Job drawing, mm, ordinate dimensions from the low corner. One solid piece. A direction names the side the tool comes from. Give positions to 0.01 mm unless a question says otherwise; leave off trailing zeros. Write each loop counter-clockwise with the first axis right and the second up, starting at its lowest first coordinate (ties: lowest second). Pieces come first, ordered by that corner, then holes. Notation, with made-up numbers: (53, 22) - (73, 22) arc R35 cw to (73, 56) - close; hole circle Ø1 at (5, 24). An arc over 180 degrees is marked (long way). Put each result on its own line as item: value. Start each with the question number.
1. Mould opens along X. For the marked faces 3, 4 and 5 say: +X half, -X half, draft (parallel to the pull), parting line (faces both ways), or undercut.
2. Cut at D-D on y = 44. List the corners of the cut face in (x, z), and give its area (3 significant figures).
3. Drop flat-ended pins along their axis: pin 1 (20.5 mm diameter, centred on x = 33.5, y = 49, fed in from +Z); pin 2 (12.5 mm diameter, centred on x = 43, z = 24, fed in from -Y). Give the stop position or say it passes through.
4. Wall check: line 1 (X direction, y = 45.5, z = 72); line 2 (Z direction, x = 50, y = 72). Give the ranges that are in metal, low to high.
5. Cut at A-A on z = 48. List the corners of the cut face in (x, y).
6. Tool access for the marked faces 1 and 2: list every direction of +Z, -Z, +X, -X, +Y, -Y with a clear straight run to the whole face (end or side of a thin tool).
7. Cut at C-C on z = 18. List the corners of the cut face in (x, y).
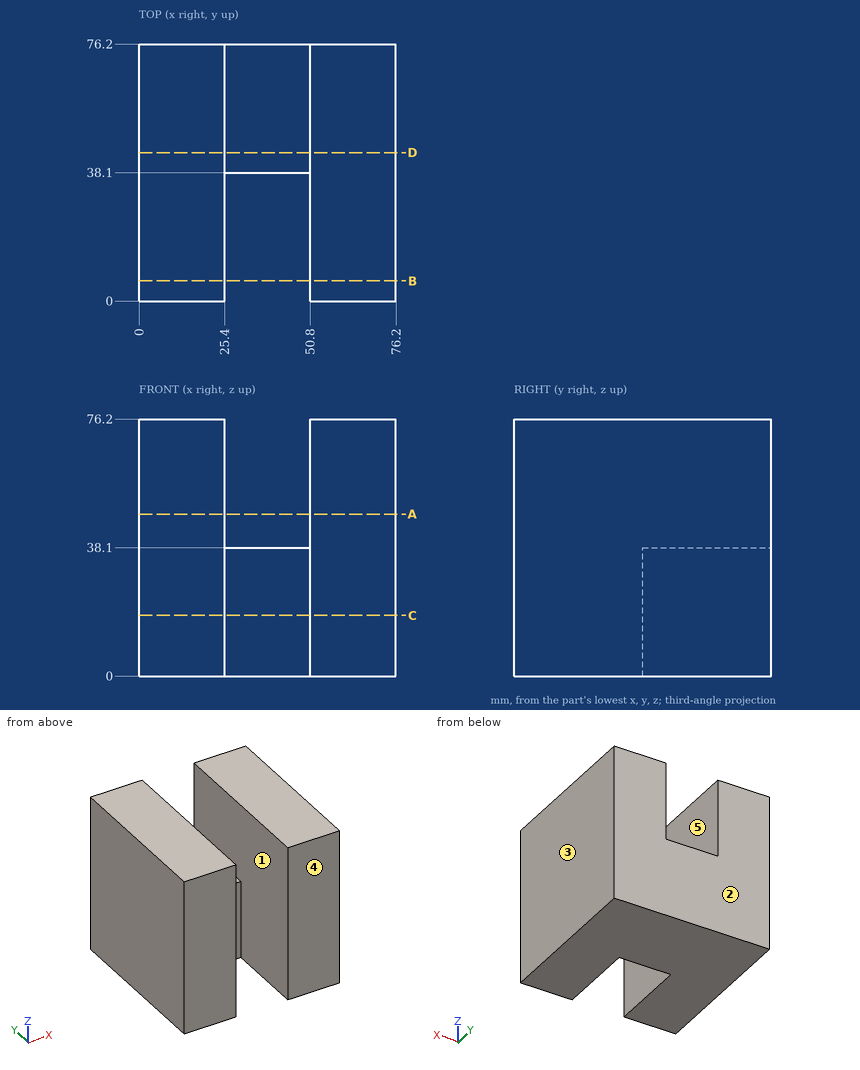
Report:
1. face 3: +X half
1. face 4: draft
1. face 5: undercut
2. outline: (0, 0) - (76.2, 0) - (76.2, 76.2) - (50.8, 76.2) - (50.8, 38.1) - (25.4, 38.1) - (25.4, 76.2) - (0, 76.2) - close
2. area: 4,840 mm²
3. pin 1: stops at z = 76.2
3. pin 2: stops at y = 38.1
4. line 1: x = 0 to 25.4, 50.8 to 76.2
4. line 2: z = 0 to 38.1
5. outline: (0, 0) - (25.4, 0) - (25.4, 76.2) - (0, 76.2) - close; (50.8, 0) - (76.2, 0) - (76.2, 76.2) - (50.8, 76.2) - close
6. face 1: +Z, -Y
6. face 2: +Z, -Z, +X, -X, +Y
7. outline: (0, 0) - (25.4, 0) - (25.4, 38.1) - (50.8, 38.1) - (50.8, 0) - (76.2, 0) - (76.2, 76.2) - (0, 76.2) - close
